Could you check a few things on this drawing? It's one solid part, dimensions in mm from its lowest x, y, z. Give positions to 0.01 mm unless a question says otherwise; leave off trailing zeros. Loops run counter-clockwise (first coordinate to the right, second up) from the corner with the lowest first, then second, coordinate; pieces in that order, holes last. Notation, with made-up numbers: M -39.5,89.5 L -29.5,89.5 A32 cw -29.5,118.5 Z; hole C 42.25,-35 d2. An arc over 180 degrees is marked long. Write each question's results on one line, items separated by ' | '. Start each with the question number.
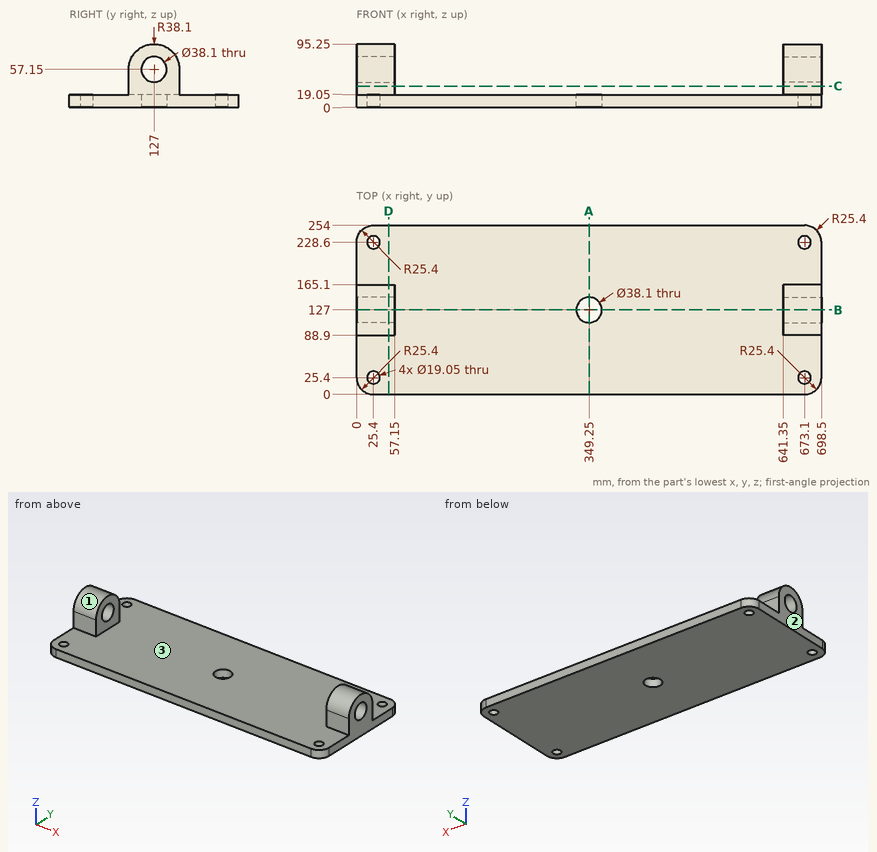
1) If we section it at A-A on x = 349.25: Write out the boundary of the cut face in (y, z).
2) I'm going to push flat-ended pins straight in: P1, Ø11.5, axis at x = 681.5, z = 36, coming from the +Y side; P2, Ø22, axis at x = 25.4, y = 228.6, coming from the +Z side. Where does each tip first touch, or does it pass through?
3) If we section it at D-D on x = 48: Write out the boundary of the cut face in (y, z).
4) If we section it at B-B on y = 127: Write out the boundary of the cut face in (x, z), plus the area to 3 significant figures.
5) If we section it at C-C on z = 32: Write out the boundary of the cut face in (x, y).
6) Please list where these lines run through material, in increasing order: line 1 (Y direction, x = 25.4, z = 11.25) (3 decimals); line 2 (X direction, y = 105, z = 24); line 3 (Z direction, x = 582.5, y = 242.5). Write a range as from..to.
7) Thinking about a two-plate mould opening in X: for the marked faces 1, 2 and 3, which applies, pulls with the +X half, pulls with the -X half, needs draft (parallel to the pull), parting line crosses it, or undercut?
Calculated:
1) outline: M 0,0 L 107.95,0 L 107.95,19.05 L 0,19.05 Z; M 146.05,0 L 254,0 L 254,19.05 L 146.05,19.05 Z
2) P1: stops at y = 165.1 | P2: stops at z = 19.05
3) outline: M 0,0 L 254,0 L 254,19.05 L 165.1,19.05 L 165.1,57.15 A38.1 ccw 88.9,57.15 L 88.9,19.05 L 0,19.05 Z; hole C 127,57.15 d38.1
4) outline: M 0,0 L 330.2,0 L 330.2,19.05 L 57.15,19.05 L 57.15,38.1 L 0,38.1 Z; M 0,76.2 L 57.15,76.2 L 57.15,95.25 L 0,95.25 Z; M 368.3,0 L 698.5,0 L 698.5,38.1 L 641.35,38.1 L 641.35,19.05 L 368.3,19.05 Z; M 641.35,76.2 L 698.5,76.2 L 698.5,95.25 L 641.35,95.25 Z | area: 16,900 mm2
5) outline: M 0,88.9 L 57.15,88.9 L 57.15,165.1 L 0,165.1 Z; M 641.35,88.9 L 698.5,88.9 L 698.5,165.1 L 641.35,165.1 Z
6) line 1: y = 0..15.875, 34.925..219.075, 238.125..254 | line 2: x = 0..57.15, 641.35..698.5 | line 3: z = 0..19.05
7) face 1: needs draft | face 2: pulls with the -X half | face 3: undercut
